from build123d import *

# Parameters (mm, degrees)
F0_R     = 76.2
F0_R_2   = 73.025
F1_DEPTH = 355.6
F2_R     = 76.2
F2_R_2   = 57.15
F3_DEPTH = 3.175
F4_R     = 3.3782
F5_DEPTH = 358.776
F7_R     = 22.225
F8_DEPTH = 7.6392352968


with BuildPart() as f1:
    # F0 (on Right) → F1 (new body)
    with BuildSketch(Plane.YZ):
        Circle(F0_R)
        Circle(F0_R_2, mode=Mode.SUBTRACT)
    extrude(amount=-F1_DEPTH)

    # F2 (on Right) → F3 (join)
    with BuildSketch(Plane.YZ):
        Circle(F2_R)
        Circle(F2_R_2, mode=Mode.SUBTRACT)
    extrude(amount=F3_DEPTH)

    # F4 (on face) → F5 (cut, through all)
    with BuildSketch(Plane.YZ.offset(3.175)):
        with Locations((0, 65.0875)):
            Circle(F4_R)
        with Locations((32.54375, 56.3674284688)):
            Circle(F4_R)
        with Locations((56.3674284688, 32.54375)):
            Circle(F4_R)
        with Locations((65.0875, 0)):
            Circle(F4_R)
        with Locations((56.3674284688, -32.54375)):
            Circle(F4_R)
        with Locations((32.54375, -56.3674284688)):
            Circle(F4_R)
        with Locations((0, -65.0875)):
            Circle(F4_R)
        with Locations((-32.54375, -56.3674284688)):
            Circle(F4_R)
        with Locations((-56.3674284688, -32.54375)):
            Circle(F4_R)
        with Locations((-65.0875, 0)):
            Circle(F4_R)
        with Locations((-56.3674284688, 32.54375)):
            Circle(F4_R)
        with Locations((-32.54375, 56.3674284688)):
            Circle(F4_R)
    extrude(amount=-F5_DEPTH, mode=Mode.SUBTRACT)

    # F7 (on offset) → F8 (cut, up to face)
    with BuildSketch(Plane.XZ.offset(76.2)):
        with Locations((-50.8, 0)):
            Circle(F7_R)
    extrude(amount=-F8_DEPTH, mode=Mode.SUBTRACT)


solid = f1.part
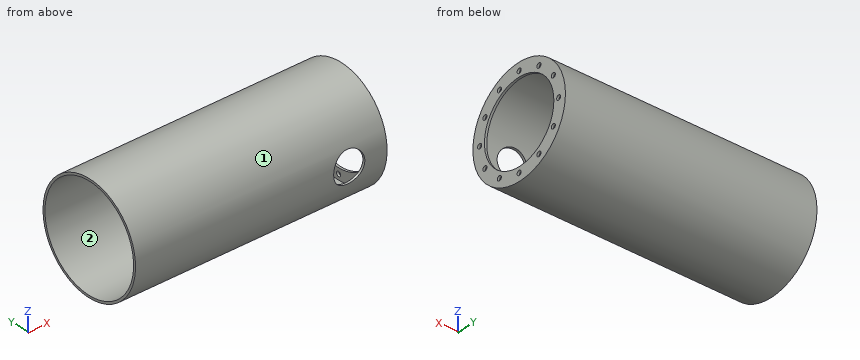
Part model, mm, in its own coordinate system. Face numbers are marked on the shaded views. Coordinates: 2 decimals unless noted, no trailing zeros. Loops run counter-clockwise (first coordinate to the right, second up) from the corner with the lowest first, then second, coordinate; pieces in that order, holes last. Notation, with made-up numbers: M -25.5,54.25 L 19.5,54.25 A14 ccw 19.5,69.25 Z; hole C 24.5,57.5 d9. An arc over 180 degrees is marked long. Use a Markdown table: item, result. Add a question column.
Q1. Cut at D-D (x = -137). Write the cut outline in (y, z) (3 decimals).
Q2. Cut at C-C (y = -47). Write the cut outline in (x, z) (3 decimals).
Q3. Mould opens along Y. For the marked faces 1 and 2 say: +Y half, -Y half, draft (parallel to the pull), parting line (faces both ways), or undercut.
Q4. Cut at B-B (y = 0). Write the cut outline in (x, z) (3 decimals), and give its area (3 significant figures).
Q5. Probe L1, parallel to Z at x = 2.35, y = 0; L2, parallel to Z at x = -180, y = 3; L3, parallel to Y at x = -137, z = -53.5. List the from-to ranges inside material, lowest first.
Q6. Pin check, flat tips, straight feed: P1, Ø1.5, axis at x = -203, y = 57, coming from the +Z side; P2, Ø9, axis at y = -56.37, z = 32.54, coming from the -X side; P3, Ø6, axis at x = -172, z = 32.5, coming from the -Y side. Stop position of each tip, or through.
Q7. Cut at A-A (z = 0). Write the cut outline in (x, y) (3 decimals), and give its area (4 significant figures).
Worked out:
| question | item | result |
|---|---|---|
| 1 | outline | C 0,0 d152.4; hole C 0,0 d146.05 |
| 2 | outline | M -355.6,-59.979 L 3.175,-59.979 L 3.175,-32.513 L 0,-32.513 L 0,-55.89 L -355.6,-55.89 Z; M -355.6,55.89 L 0,55.89 L 0,32.513 L 3.175,32.513 L 3.175,59.979 L -355.6,59.979 Z |
| 3 | face 1 | parting line |
| 3 | face 2 | undercut |
| 4 | outline | M -355.6,-76.2 L 3.175,-76.2 L 3.175,-68.466 L 0,-68.466 L 0,-73.025 L -355.6,-73.025 Z; M -355.6,73.025 L 0,73.025 L 0,68.466 L 3.175,68.466 L 3.175,76.2 L -355.6,76.2 Z; M 0,-61.709 L 3.175,-61.709 L 3.175,-57.15 L 0,-57.15 Z; M 0,57.15 L 3.175,57.15 L 3.175,61.709 L 0,61.709 Z |
| 4 | area | 2,340 mm2 |
| 5 | L1 | z = -76.2 to -68.47, -61.71 to -57.15, 57.15 to 61.71, 68.47 to 76.2 |
| 5 | L2 | z = -76.14 to -72.96, 72.96 to 76.14 |
| 5 | L3 | y = -54.26 to -49.7, 49.7 to 54.26 |
| 6 | P1 | stops at z = 51.4 |
| 6 | P2 | stops at x = 0 |
| 6 | P3 | stops at y = -70.26 |
| 7 | outline | M -355.6,-76.2 L -73.025,-76.2 L -73.025,-73.025 L -355.6,-73.025 Z; M -355.6,73.025 L 0,73.025 L 0,68.466 L 3.175,68.466 L 3.175,76.2 L -355.6,76.2 Z; M -28.575,-76.2 L 3.175,-76.2 L 3.175,-68.466 L 0,-68.466 L 0,-73.025 L -28.575,-73.025 Z; M 0,-61.709 L 3.175,-61.709 L 3.175,-57.15 L 0,-57.15 Z; M 0,57.15 L 3.175,57.15 L 3.175,61.709 L 0,61.709 Z |
| 7 | area | 2,195 mm2 |
